from build123d import *

# Parameters (mm, degrees)
F0_R     = 1.5
F1_DEPTH = 3


with BuildPart() as f1:
    # F0 (on Front) → F1 (new body)
    with BuildSketch(Plane.XZ):
        Polygon((2, 39), (2, 42), (-4, 42), (-4, -42), (2, -42), (2, -39), (4, -39), (4, -31), (2, -31), (2, -28), (4, -28), (4, 22), (2, 22), (2, 25), (4, 25), (4, 39), align=None)
        with Locations((-1, -33)):
            Circle(F0_R, mode=Mode.SUBTRACT)
        with Locations((-1, 27)):
            Circle(F0_R, mode=Mode.SUBTRACT)
    extrude(amount=F1_DEPTH)


solid = f1.part
CAD build for the part. Positions are in the model's coordinates, mm. A direction names the side the tool comes from. Give positions to 0.01 mm unless a question says otherwise; leave off trailing zeros. Write each loop counter-clockwise with the first axis right and the second up, starting at its lowest first coordinate (ties: lowest second). Pieces come first, ordered by that corner, then holes. Notation, with made-up numbers: (70.5, -36.75) -> (107.5, -36.75) arc R17 cw to (107.5, -27.75) -> close; hole circle Ø4 at (76, -30.5). An arc over 180 degrees is marked (long way). Return JSON: item names as keys, results as strings.
Item 1: Drop flat-ended pins along their axis: pin 1 (0.6 mm diameter, centred on x = 3, y = -2, fed in from -Z); pin 2 (1.6 mm diameter, centred on x = 3.5, y = -1, fed in from +Z); pin 3 (2.5 mm diameter, centred on x = -1, z = -33, fed in from -Y); pin 4 (0.9 mm diameter, centred on y = -1.5, z = -40.5, fed in from +X). Give the stop position or say it passes through.
Answer below:
{"pin 1": "stops at z = -39", "pin 2": "stops at z = 39", "pin 3": "passes through", "pin 4": "stops at x = 2"}
Item 2: Band-saw the part on B-B (x = -1). List the corners of the cut face in (y, z), then the cut area to 3 significant figures.
Answer below:
{"outline": "(-3, -42) -> (0, -42) -> (0, -34.5) -> (-3, -34.5) -> close; (-3, -31.5) -> (0, -31.5) -> (0, 25.5) -> (-3, 25.5) -> close; (-3, 28.5) -> (0, 28.5) -> (0, 42) -> (-3, 42) -> close", "area": "234 mm2"}
Item 3: Band-saw the part on C-C (y = -0.5). List the corners of the cut face in (x, z).
Answer below:
{"outline": "(-4, -42) -> (2, -42) -> (2, -39) -> (4, -39) -> (4, -31) -> (2, -31) -> (2, -28) -> (4, -28) -> (4, 22) -> (2, 22) -> (2, 25) -> (4, 25) -> (4, 39) -> (2, 39) -> (2, 42) -> (-4, 42) -> close; hole circle Ø3 at (-1, -33); hole circle Ø3 at (-1, 27)"}
Item 4: Two-plate mould, pull along Z, no slides. Class faces 5 (the cylindrical face through (-1.195, -1.479, 28.487)), 6 (the flat face through (4, -1, 32)), 7 (the flat face through (3, -1, 39)): +Z half, -Z half, draft (parallel to the pull), parting line (faces both ways), or undercut.
Answer below:
{"face 5": "undercut", "face 6": "draft", "face 7": "+Z half"}
Item 5: Drill centre lines: probe 1 along Z at (x, y) = (-1, -1.7); probe 2 along Z at (x, y) = (3, -1.9). Where is each one in solid material? Low to high.
Answer below:
{"probe 1": "z = -42 to -34.5, -31.5 to 25.5, 28.5 to 42", "probe 2": "z = -39 to -31, -28 to 22, 25 to 39"}
Item 6: Tool access for faces 1 (the flat face through (3, -1, -31)), 2 (the flat face through (4, -1, -3)), 3 (the flat face through (2, -1, 40)), 4 (the flat face through (2, -1, -41)): list every direction of +Z, -Z, +X, -X, +Y, -Y with a clear straight run to the whole face (end or side of a thin tool).
Answer below:
{"face 1": "+X, +Y, -Y", "face 2": "+Z, -Z, +X, +Y, -Y", "face 3": "+Z, +X, +Y, -Y", "face 4": "-Z, +X, +Y, -Y"}
Item 7: Band-saw the part on A-A (z = -33). List the corners of the cut face in (x, y), then the cut area to 3 significant figures.
Answer below:
{"outline": "(-4, -3) -> (-2.5, -3) -> (-2.5, 0) -> (-4, 0) -> close; (0.5, -3) -> (4, -3) -> (4, 0) -> (0.5, 0) -> close", "area": "15.0 mm2"}
